Input: part model. Units: mm. Frame: model coordinates. Coordinates: 2 decimals unless noted, no trailing zeros. Write each loop counter-clockwise with the first axis right and the second up, starting at its lowest first coordinate (ties: lowest second). Pieces come first, ordered by that corner, then holes. Notation, with made-up numbers: M 14.5,-20.5 L 32.5,-20.5 A24 cw 32.5,2.5 Z; hole C 78.5,5 d7. An arc over 180 degrees is marked long. Use one line per item in the form item = value.
from build123d import *

# Parameters (mm, degrees)
BOSS_EXTRUDE1_DEPTH = 5.08
SKETCH2_R           = 0.35
BOSS_EXTRUDE2_DEPTH = 3.38


with BuildPart() as part:
    # Sketch1 → Boss-Extrude1 (new body)
    with BuildSketch(Plane(origin=(0, 0, 0), x_dir=(1, 0, 0), z_dir=(0, 1, 0))):
        Polygon((-1.016, -1.016), (0.254, -2.286), (2.286, -2.286), (3.556, -1.016), (3.556, 1.016), (-1.016, 1.016), align=None)
    extrude(amount=BOSS_EXTRUDE1_DEPTH)

    # Sketch2 → Boss-Extrude2 (add)
    with BuildSketch(Plane.XZ):
        Circle(SKETCH2_R)
        with Locations((1.27, 0)):
            Circle(SKETCH2_R)
        with Locations((2.54, 0)):
            Circle(SKETCH2_R)
    extrude(amount=BOSS_EXTRUDE2_DEPTH)


solid = part.part
(1) Section query D-D on z = -0.7. Return the cut outline in (x, y), plus the area to 3 significant figures.
Computed:
outline = M -1.02,0 L 3.56,0 L 3.56,5.08 L -1.02,5.08 Z
area = 23.2 mm^2
(2) Section query C-C on y = -1. Return the cut outline in (x, z), plus the area to 3 significant figures.
Computed:
outline = C 0,0 d0.7; C 1.27,0 d0.7; C 2.54,0 d0.7
area = 1.15 mm^2
(3) Section query B-B on x = 1.4. Return the cut outline in (y, z), plus the area to 3 significant figures.
Computed:
outline = M -3.38,-0.32 L 0,-0.32 L 0,-1.02 L 5.08,-1.02 L 5.08,2.29 L 0,2.29 L 0,0.32 L -3.38,0.32 Z
area = 19.0 mm^2
(4) Section query A-A on y = 1.5. Return the cut outline in (x, z), plus the area to 3 significant figures.
Computed:
outline = M -1.02,-1.02 L 3.56,-1.02 L 3.56,1.02 L 2.29,2.29 L 0.25,2.29 L -1.02,1.02 Z
area = 13.5 mm^2
(5) Line query: probe 1 along X at (y, z) = (-0.5, 0.2); probe 2 along Y at (x, z) = (1.8, -0.4); probe 3 along Z at (x, y) = (0, -0.25). Output: solid intervals per line, ascending.
Computed:
probe_1 = -0.29 to 0.29, 0.98 to 1.56, 2.25 to 2.83
probe_2 = 0 to 5.08
probe_3 = -0.35 to 0.35
